Check sheet for the modelled part. Datum: model origin and axes. Units: mm. Face numbers are marked on the shaded views. Round coordinates to 2 decimals unless told otherwise and drop trailing zeros. Loops run counter-clockwise (first coordinate to the right, second up) from the corner with the lowest first, then second, coordinate; pieces in that order, holes last. Notation, with made-up numbers: (-15, 30) - (26, 30) arc R16 cw to (26, 40) - close; hole circle Ø9 at (39, 29). An arc over 180 degrees is marked (long way). Put each result on its own line as item: value. Start each with the question number.
```python
from build123d import *

# Parameters (mm, degrees)
SKETCH1_W           = 1.5875
SKETCH1_H           = 6.5
SKETCH1_W_2         = 10.9125
SKETCH1_H_2         = 1.5875
BOSS_EXTRUDE1_DEPTH = 6
SKETCH2_R           = 1.25
CUT_EXTRUDE1_DEPTH  = 6
SKETCH3_R           = 1.25
CUT_EXTRUDE2_DEPTH  = 6


with BuildPart() as part:
    # Sketch1 → Boss-Extrude1 (new body)
    with BuildSketch(Plane.XY):
        with Locations((0.41275, -0.74175)):
            Rectangle(SKETCH1_W, SKETCH1_H)
        with Locations((6.66275, 1.7145)):
            Rectangle(SKETCH1_W_2, SKETCH1_H_2)
    extrude(amount=BOSS_EXTRUDE1_DEPTH)

    # Sketch2 → Cut-Extrude1 (cut)
    with BuildSketch(Plane(origin=(1.2065, 0, 0), x_dir=(0, 0, -1), z_dir=(1, 0, 0))):
        with Locations(Location((-3, -1.5355, 0), (0, 0, 90))):
            Circle(SKETCH2_R)
    extrude(amount=-CUT_EXTRUDE1_DEPTH, mode=Mode.SUBTRACT)

    # Sketch3 → Cut-Extrude2 (cut)
    with BuildSketch(Plane.XZ.offset(-0.92075)):
        with Locations(Location((9.579, 3, 0), (0, 0, 270))):
            Circle(SKETCH3_R)
    extrude(amount=-CUT_EXTRUDE2_DEPTH, mode=Mode.SUBTRACT)


solid = part.part
```
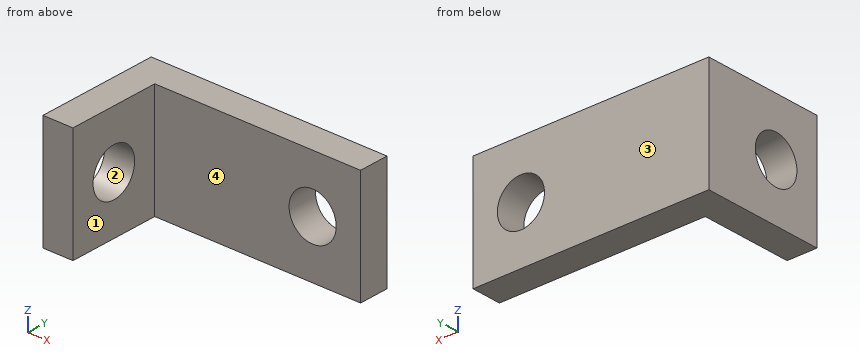
Q1. Cross-section at A-A on z = 3. Enter the section's corners in (x, y).
Q2. Cross-section at C-C on y = -2.25. Enter the section's corners in (x, z), and give its area (3 significant figures).
Q3. Draft check along Y on the marked faces 1, 2, 3 and 4. Enter one of: +Y half, -Y half, draft (parallel to the pull), parting line (faces both ways), or undercut.
Q4. Cross-section at D-D on x = 9. Enter the section's corners in (y, z), and give its area (3 significant figures).
Q5. Cross-section at B-B on x = 1. Enter the section's corners in (y, z), and give its area (3 significant figures).
Q6. Depth check by flat-ended pin: pin 1 Ø2 at (y, z) = (-1.54, 3) entering from +X; pin 2 Ø2 at (x, y) = (1, 0) entering from -Z. Enter the tip coordinate at first touch or a pass-through.
Q7. Material ranges on line 1 (X direction, y = 1.6, z = 3); line 2 (Y direction, x = 1.25, z = 5.7); line 3 (X direction, y = -0.5, z = 0.35), recorded low to high. Write a range as from..to.
Answer list:
1. outline: (-0.38, -3.99) - (1.21, -3.99) - (1.21, -2.79) - (-0.38, -2.79) - close; (-0.38, -0.29) - (1.21, -0.29) - (1.21, 0.92) - (8.33, 0.92) - (8.33, 2.51) - (-0.38, 2.51) - close; (10.83, 0.92) - (12.12, 0.92) - (12.12, 2.51) - (10.83, 2.51) - close
2. outline: (-0.38, 0) - (1.21, 0) - (1.21, 1.97) - (-0.38, 1.97) - close; (-0.38, 4.03) - (1.21, 4.03) - (1.21, 6) - (-0.38, 6) - close
2. area: 6.27 mm2
3. face 1: draft
3. face 2: undercut
3. face 3: +Y half
3. face 4: -Y half
4. outline: (0.92, 0) - (2.51, 0) - (2.51, 1.89) - (0.92, 1.89) - close; (0.92, 4.11) - (2.51, 4.11) - (2.51, 6) - (0.92, 6) - close
4. area: 6.01 mm2
5. outline: (-3.99, 0) - (2.51, 0) - (2.51, 6) - (-3.99, 6) - close; hole circle Ø2.5 at (-1.54, 3)
5. area: 34.1 mm2
6. pin 1: passes through
6. pin 2: stops at z = 0
7. line 1: x = -0.38..8.33, 10.83..12.12
7. line 2: y = 0.92..2.51
7. line 3: x = -0.38..1.21
